Work out the finished part from the listing and answer in its coordinate system (mm). A direction names the side the tool comes from. Coordinates: 2 decimals unless noted, no trailing zeros. Loops run counter-clockwise (first coordinate to the right, second up) from the corner with the lowest first, then second, coordinate; pieces in that order, holes last. Notation, with made-up numbers: (87.5, 75.5) -> (98.5, 75.5) arc R28 ccw to (98.5, 106.5) -> close; hole circle Ø6 at (7, 73.25). An arc over 180 degrees is marked (long way). Use a Markdown table: item, result. Add a question column.
```python
from build123d import *

# Parameters (mm, degrees)
SKETCH1_R           = 6
BOSS_EXTRUDE1_DEPTH = 2
SKETCH2_R           = 0.7
CUT_EXTRUDE1_DEPTH  = 0.5
SKETCH3_R           = 3
CUT_EXTRUDE2_DEPTH  = 0.5
SKETCH5_R           = 2
SKETCH4_R           = 2.5


with BuildPart() as part:
    # Sketch1 → Boss-Extrude1 (new body)
    with BuildSketch(Plane(origin=(0, 0, 0), x_dir=(0, 0, -1), z_dir=(1, 0, 0))):
        Circle(SKETCH1_R)
    extrude(amount=BOSS_EXTRUDE1_DEPTH)

    # Sketch2 → Cut-Extrude1 (cut)
    with BuildSketch(Plane.ZY):
        Circle(SKETCH2_R)
    extrude(amount=-CUT_EXTRUDE1_DEPTH, mode=Mode.SUBTRACT)

    # Sketch3 → Cut-Extrude2 (cut)
    with BuildSketch(Plane(origin=(2, 0, 0), x_dir=(0, 0, -1), z_dir=(1, 0, 0))):
        Circle(SKETCH3_R)
    extrude(amount=-CUT_EXTRUDE2_DEPTH, mode=Mode.SUBTRACT)

    # Sketch5 → Loft1 section 0
    with BuildSketch(Plane(origin=(2, 0, 0), x_dir=(0, 0, -1), z_dir=(1, 0, 0))):
        Circle(SKETCH5_R)
    # Sketch4 → Loft1 section 1
    with BuildSketch(Plane(origin=(1.5, 0, 0), x_dir=(0, 0, -1), z_dir=(1, 0, 0))):
        Circle(SKETCH4_R)
    loft()


solid = part.part
```
Item 1: Section B-B (z = 0) is taken. Determine the outline of the cut face in (x, y), then the cut area to 4 significant figures.
Item 2: For a pull along Z with two mould halves and no side action, classify faces 4 (the face through (0.2, 0, -0.7)), 5 (the face through (1, 0, 6)), 6 (the face through (2, -1, 3)) as +Z half, -Z half, draft (parallel to the pull), parting line (faces both ways), or undercut.
Item 3: Section C-C (x = 0.9) is taken. Determine the outline of the cut face in (y, z), then the cut area to 3 significant figures.
Item 4: Given pin 1 (1.1 mm diameter, centred on y = 0, z = 0.5, fed in from -X), flat-ended and moving along its own axis, determine where the tip first touches the part or whether it passes through.
Item 5: For faces 1 (the face through (0.5, 0, 0)), 2 (the face through (2, 0, 0)), 3 (the face through (1.5, 2, 2)), determine the directions among +Z, -Z, +X, -X, +Y, -Y from which every point of the face is accessible in a straight line to the end or side of a thin tool.
Item 6: Section A-A (x = 1.8) is taken. Determine the outline of the cut face in (y, z).
Item 7: Find the intervals of material crossed by probe 1 along Y at (x, z) = (1.65, 0); probe 2 along Y at (x, z) = (1.85, 0); probe 3 along Y at (x, z) = (0.35, 0), in increasing order.
Item 8: Section D-D (z = 2.75) is taken. Determine the outline of the cut face in (x, y).
Output:
| question | item | result |
|---|---|---|
| 1 | outline | (0, -6) -> (2, -6) -> (2, -3) -> (1.5, -3) -> (1.5, -2.5) -> (2, -2) -> (2, 2) -> (1.5, 2.5) -> (1.5, 3) -> (2, 3) -> (2, 6) -> (0, 6) -> (0, 0.7) -> (0.5, 0.7) -> (0.5, -0.7) -> (0, -0.7) -> close |
| 1 | area | 22.55 mm2 |
| 2 | face 4 | undercut |
| 2 | face 5 | parting line |
| 2 | face 6 | draft |
| 3 | outline | circle Ø12 at (0, 0) |
| 3 | area | 113 mm2 |
| 4 | pin 1 | stops at x = 0 |
| 5 | face 1 | -X |
| 5 | face 2 | +Z, -Z, +X, +Y, -Y |
| 5 | face 3 | +X |
| 6 | outline | circle Ø12 at (0, 0); circle Ø4.4 at (0, 0); hole circle Ø6 at (0, 0) |
| 7 | probe 1 | y = -6 to -3, -2.35 to 2.35, 3 to 6 |
| 7 | probe 2 | y = -6 to -3, -2.15 to 2.15, 3 to 6 |
| 7 | probe 3 | y = -6 to -0.7, 0.7 to 6 |
| 8 | outline | (0, -5.33) -> (2, -5.33) -> (2, -1.2) -> (1.5, -1.2) -> (1.5, 1.2) -> (2, 1.2) -> (2, 5.33) -> (0, 5.33) -> close |
